Here's how the part is built. I have some questions about the finished solid (model axes, mm). Face numbers are marked on the shaded views. A direction names the side the tool comes from. Give positions to 0.01 mm unless a question says otherwise; leave off trailing zeros. Loops run counter-clockwise (first coordinate to the right, second up) from the corner with the lowest first, then second, coordinate; pieces in that order, holes last. Notation, with made-up numbers: M 82,38.25 L 121,38.25 A28 cw 121,64.25 Z; hole C -4.5,-18 d1. An arc over 180 degrees is marked long. Answer as CSV lines item,"result". Start each with the question number.
Item 1: For the marked faces 1 and 2, which set-ups out of +Z, -Z, +X, -X, +Y, -Y let a thin tool reach every point of the face, with its end or its side?
Item 2: If I drill on line 1 along X through (y, z) = (16, 5.25); line 2 along X through (y, z) = (6.75, 8.75); line 3 along Y through (x, z) = (9, 14), over which ranges is the centre line in solid material (lowest first)? Write a range as from..to.
Item 3: I want a section at D-D on z = 3. List the corners of the cut face in (x, y) for me, plus the area to 3 significant figures.
Item 4: I want a section at A-A on z = 7.5. List the corners of the cut face in (x, y) for me, plus the area to 3 significant figures.
Item 5: I want a section at B-B on y = 13. List the corners of the cut face in (x, z) for me.
Item 6: Will these pins go through, and if not, where does the flat tip stop? P1, Ø4, axis at x = -5.5, z = 12, coming from the -Y side; P2, Ø1.1, axis at y = 25.5, z = 9, coming from the -X side; P3, Ø0.8, axis at y = 25, z = 5, coming from the +X side.
Item 7: I want a section at C-C on x = -12.5. List the corners of the cut face in (y, z) for me, plus the area to 3 significant figures.
Item 8: If we mould it in two halves opening along X, with no side actions, what happens to the marked faces 3, 4 and 5? For each: released by +X, released by -X, zero draft, split by the parting line, or undercut.
Autodesk Inventor part; units mm, degrees
ref_plane "YZ Plane" through (0, 0, 0) normal (1, 0, 0) x (0, 1, 0)
ref_plane "XZ Plane" through (0, 0, 0) normal (0, 1, 0) x (-1, 0, 0)
ref_plane "XY Plane" through (0, 0, 0) normal (0, 0, 1) x (1, 0, 0)
sketch "Sketch1" plane through (0, 0, 0) normal (0, 0, 1) x (1, 0, 0)
  line L0 (0, 0) -> (-34.45, 0)
  line L1 (-34.45, 0) -> (-34.45, 25.6)
  line L2 (-34.45, 25.6) -> (-32.15, 25.6)
  line L3 (-32.15, 25.6) -> (-32.15, 24.6)
  line L4 (-32.15, 24.6) -> (-32.95, 24.6)
  line L5 (-32.95, 24.6) -> (-32.95, 23)
  line L6 (-32.95, 23) -> (-32.15, 23)
  line L7 (-32.15, 23) -> (-32.15, 3)
  line L8 (-32.15, 3) -> (0, 3)
  line L9 (0, 3) -> (0, 0)
  point P0 (-32.95, 23.8)
  point P1 (0, 1.5)
  dimension "d0" = 3
  dimension "d2" = 0.8
  dimension "d3" = 1
  dimension "d4" = 1.6
  dimension "d5" = 1.5
  dimension "d9" = 20
  dimension "d15" = 65.9
extrude "Extrusion1" add sketch "Sketch1" along normal blind 15
mirror "Mirror1" about plane through (0, 0, 0) normal (1, 0, 0) of "Extrusion1"
sketch "Sketch2" plane through (-32.15, 3, 15) normal (0, 1, 0) x (1, 0, 0)
  line L0 (64.3, 15) -> (0, 15) construction
  line L1 (0, 15) -> (0, 0) construction
  line L2 (0, 0) -> (64.3, 0) construction
  line L3 (64.3, 15) -> (64.3, 0) construction
  line L4 (15.5721, 7.5) -> (48.7279, 7.5) construction
  line L5 (15.5721, 5.3) -> (48.7279, 5.3)
  line L6 (48.7279, 9.7) -> (15.5721, 9.7)
  arc A0 (15.5721, 9.7) -> (15.5721, 5.3) centre (15.5721, 7.5) ccw
  arc A1 (48.7279, 5.3) -> (48.7279, 9.7) centre (48.7279, 7.5) ccw
  line L7 (66.6, 15) -> (66.6, 0)
  point P0 (32.15, 15)
  point P1 (32.15, 7.5)
  point P2 (32.15, 15)
  point P3 (66.6, 7.5)
  dimension "d12" = 2.2
extrude "Extrusion2" cut sketch "Sketch2" against normal through all
chamfer "Chamfer1" distance 1.5 angle 45 2 edges at (-34.45, 25.6, 7.5) (34.45, 25.6, 7.5)
fillet "Fillet1" radius 4 2 edges at (32.15, 3, 7.5) (-32.15, 3, 7.5)
properties part number "Discovery boar clamp"
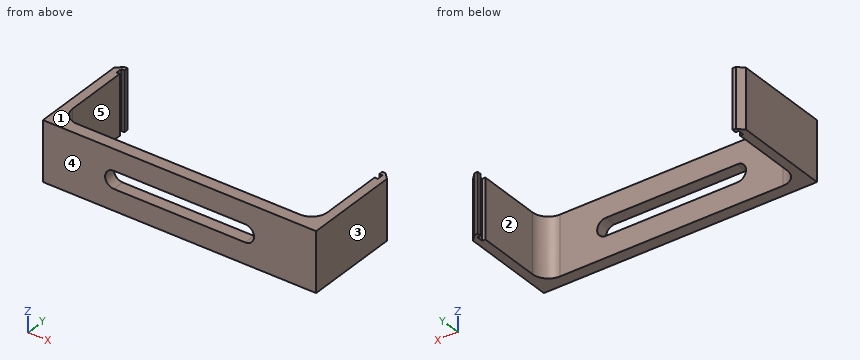
Result:
1,face 1,"+Z, +X, -X, +Y, -Y"
1,face 2,"+Z, -Z, +Y"
2,line 1,"-34.45..-32.15, 32.15..34.45"
2,line 2,"-34.45..-32.14, 32.14..34.45"
2,line 3,"0..3"
3,outline,"M -34.45,0 L 34.45,0 L 34.45,24.1 L 32.95,25.6 L 32.15,25.6 L 32.15,24.6 L 32.95,24.6 L 32.95,23 L 32.15,23 L 32.15,7 A4 cw 28.15,3 L -28.15,3 A4 cw -32.15,7 L -32.15,23 L -32.95,23 L -32.95,24.6 L -32.15,24.6 L -32.15,25.6 L -32.95,25.6 L -34.45,24.1 Z"
3,area,"313 mm^2"
4,outline,"M -34.45,0 L -18.78,0 L -18.78,3 L -28.15,3 A4 cw -32.15,7 L -32.15,23 L -32.95,23 L -32.95,24.6 L -32.15,24.6 L -32.15,25.6 L -32.95,25.6 L -34.45,24.1 Z; M 18.78,0 L 34.45,0 L 34.45,24.1 L 32.95,25.6 L 32.15,25.6 L 32.15,24.6 L 32.95,24.6 L 32.95,23 L 32.15,23 L 32.15,7 A4 cw 28.15,3 L 18.78,3 Z"
4,area,"200 mm^2"
5,outline,"M -34.45,0 L -32.15,0 L -32.15,15 L -34.45,15 Z; M 32.15,0 L 34.45,0 L 34.45,15 L 32.15,15 Z"
6,P1,"y = 0"
6,P2,"x = -33.6"
6,P3,"x = 33.95"
7,outline,"M 0,0 L 3,0 L 3,5.3 L 0,5.3 Z; M 0,9.7 L 3,9.7 L 3,15 L 0,15 Z"
7,area,"31.8 mm^2"
8,face 3,"released by +X"
8,face 4,"zero draft"
8,face 5,"undercut"
